Build history of the part. All positions in model axes, mm. A direction names the side the tool comes from. Give positions to 0.01 mm unless a question says otherwise; leave off trailing zeros. Loops run counter-clockwise (first coordinate to the right, second up) from the corner with the lowest first, then second, coordinate; pieces in that order, holes last. Notation, with made-up numbers: M -40,-35 L -9,-35 A29 ccw -9,1 Z; hole C 85,-31 d4. An arc over 180 degrees is marked long. Put each result on its own line as item: value.
Autodesk Inventor part; units mm, degrees
ref_plane "YZ Plane" through (0, 0, 0) normal (1, 0, 0) x (0, 1, 0)
ref_plane "XZ Plane" through (0, 0, 0) normal (0, 1, 0) x (-1, 0, 0)
ref_plane "XY Plane" through (0, 0, 0) normal (0, 0, 1) x (1, 0, 0)
sketch "Sketch1" plane through (0, 0, 0) normal (1, 0, 0) x (0, 1, 0)
  line L0 (-20.4, 45.3) -> (20.4, 45.3)
  line L1 (20.4, 45.3) -> (20.4, -45.3)
  line L2 (20.4, -45.3) -> (-20.4, -45.3)
  line L3 (-20.4, -45.3) -> (-20.4, 45.3)
  line L4 (-20.4, 45.3) -> (20.4, -45.3) construction
  line L5 (20.4, 45.3) -> (-20.4, -45.3) construction
  point P0 (0, 0)
  dimension "d0" = 40.8
  dimension "d1" = 90.6
extrude "Extrusion1" add sketch "Sketch1" along normal blind 4
sketch "Sketch2" plane through (4, 0, 0) normal (1, 0, 0) x (0, 0, -1)
  circle A0 centre (-24.3, 0) radius 16
  line L0 (-45.3, 20.4) -> (-45.3, -20.4)
  line L1 (-45.3, 0) -> (-40.3, 0)
  line L2 (-45.3, 0) -> (-41.0258, 0)
  line L3 (45.3, 20.4) -> (-45.3, 20.4)
  line L4 (-45.3, -20.4) -> (45.3, -20.4)
  circle A1 centre (24.3, 0) radius 16
  dimension "d4" = 32
extrude "Extrusion2" add sketch "Sketch2" along normal blind 24
sketch "Sketch3" plane through (4, 0, 0) normal (1, 0, 0) x (0, 0, -1)
  line L0 (-45.3, 20.4) -> (-45.3, -20.4)
  line L1 (-45.3, -20.4) -> (45.3, -20.4)
  line L2 (-45.3, 20.4) -> (45.3, -20.4)
  line L3 (45.3, -20.4) -> (45.3, 20.4)
  line L4 (-45.3, -20.4) -> (45.3, 20.4)
  circle A0 centre (0, 0) radius 5
  line L5 (0, 0) -> (0, -27.8597)
  dimension "d9" = 10
sketch "Sketch4" plane through (0, 0, 0) normal (-1, 0, 0) x (0, 0, 1)
  line L0 (-45.3, -20.4) -> (-45.3, 20.4)
  line L1 (45.3, 20.4) -> (45.3, -20.4)
  line L2 (-45.3, 20.4) -> (45.3, 20.4)
  line L3 (45.3, 20.4) -> (45.3, -20.4)
  line L4 (45.3, -20.4) -> (-45.3, -20.4)
  line L5 (-45.3, -20.4) -> (-45.3, 20.4)
  point P0 (0, 0)
scale "Scale1" factors (0.5, 0.5, 0.5) then translate (0, 0, 0) bodies 1
properties part number "Ultrasound" material "PET Plastic"
Q1. Slice it at B-B (y = 0). List the corners of the cut face in (x, z), and give its area (3 significant figures).
Here are the results:
outline: M 0,-22.65 L 2,-22.65 L 2,-20.15 L 14,-20.15 L 14,-4.15 L 2,-4.15 L 2,4.15 L 14,4.15 L 14,20.15 L 2,20.15 L 2,22.65 L 0,22.65 Z
area: 475 mm²
Q2. Mould opens along Z. For faces 1 (the flat face through (2, 0, 0)), 2 (the flat face through (14, 0, -12)), 3 (the flat face through (1, 0, -22.65)) say: pulls with the +Z half, pulls with the -Z half, needs draft (parallel to the pull), parting line crosses it, or undercut.
Here are the results:
face 1: undercut
face 2: needs draft
face 3: pulls with the -Z half
Q3. Probe line 1 (X direction, y = -9.5, z = 16.5); line 2 (Z direction, x = 2.5, y = -5.75); line 3 (Z direction, x = 10.25, y = 2.25). List the from-to ranges inside material, lowest first. Write a range as from..to.
Here are the results:
line 1: 0..2
line 2: -17.71..-6.59, 6.59..17.71
line 3: -19.83..-4.47, 4.47..19.83
Q4. Slice it at C-C (x = 3). List the corners of the cut face in (y, z).
Here are the results:
outline: C 0,-12.15 d16; C 0,12.15 d16
Q5. Tool access for faces 4 (the flat face through (14, 0, 12)), 5 (the cylindrical face through (7.92, 3.06, 4.76)): list every direction of +Z, -Z, +X, -X, +Y, -Y with a clear straight run to the whole face (end or side of a thin tool).
Here are the results:
face 4: +Z, -Z, +X, +Y, -Y
face 5: +X
Q6. Slice it at D-D (z = -11.5). List the corners of the cut face in (x, y).
Here are the results:
outline: M 0,-10.2 L 2,-10.2 L 2,-7.97 L 14,-7.97 L 14,7.97 L 2,7.97 L 2,10.2 L 0,10.2 Z
Q7. Drop flat-ended pins along their axis: pin 1 Ø6 at (x, y) = (6, -5.5) entering from +Z; pin 2 Ø5 at (x, z) = (7.5, -12) entering from -Y; pin 3 Ø4 at (x, y) = (12, -5.5) entering from +Z. Give the stop position or say it passes through.
Here are the results:
pin 1: z = 19.75
pin 2: y = -8
pin 3: z = 19.34
Q8. Slice it at A-A (z = 12.15). List the corners of the cut face in (x, y).
Here are the results:
outline: M 0,-10.2 L 2,-10.2 L 2,-8 L 14,-8 L 14,8 L 2,8 L 2,10.2 L 0,10.2 Z
